The listing builds one solid part. Answer for the finished solid, in the listing's coordinates (mm). A direction names the side the tool comes from. Round coordinates to 2 decimals unless told otherwise and drop trailing zeros. Write each loop counter-clockwise with the first axis right and the second up, starting at its lowest first coordinate (ties: lowest second). Pieces come first, ordered by that corner, then holes. Notation, with made-up numbers: M 24,-21.5 L 70,-21.5 A10 ccw 70,-17.5 Z; hole C -33,4.25 d9. An arc over 180 degrees is marked long. One line per item, written item: value. Start each with the question number.
(1) Consider probe 1 along Y at (x, z) = (0, 4.75); probe 2 along Z at (x, y) = (3, -9.25); probe 3 along X at (y, z) = (0.25, 4). Determine where each line is inside the solid, lowest interval first.
(2) Given P1, Ø1.8, axis at x = 0, y = -0.5, coming from the +Z side; P2, Ø6, axis at y = 2, z = 5.5, coming from the -X side; P3, Ø5, axis at x = -7.5, z = 4, coming from the -Y side, each flat-ended and moving along its own axis, determine where each tip first touches the part or whether it passes through.
(3) Section B-B (z = 8.75) is taken. Determine the outline of the cut face in (x, y).
(4) For faces 1 (the flat face through (-2, -3, 10.5)), 2 (the flat face through (5, 0, 2)), determine the directions among +Z, -Z, +X, -X, +Y, -Y from which every point of the face is accessible in a straight line to the end or side of a thin tool.
(5) Section A-A (y = 0) is taken. Determine the outline of the cut face in (x, z).
(6) For a pull along Y with two mould halves and no side action, classify faces 3 (the cylindrical face through (-0.867, -3.905, 6.092)), 4 (the cylindrical face through (-3, 0, 6)), 5 (the flat face through (0, 0, 0)) as released by +Y, released by -Y, zero draft, split by the parting line, or undercut.
```python
from build123d import *

# Parameters (mm, degrees)
F0_R     = 11
F1_DEPTH = 2
F2_R     = 4
F2_R_2   = 3
F3_DEPTH = 8.5
F4_R     = 0.2
F5_SIZE  = 0.2


with BuildPart() as f1:
    # F0 (on Top) → F1 (new body)
    with BuildSketch(Plane.XY):
        Circle(F0_R)
    extrude(amount=F1_DEPTH)

    # F2 (on face) → F3 (join)
    with BuildSketch(Plane.XY.offset(2)):
        Circle(F2_R)
        Circle(F2_R_2, mode=Mode.SUBTRACT)
    extrude(amount=F3_DEPTH)

    # F4
    f4_edges = [f1.edges().sort_by_distance(p)[0] for p in [
        (-4, 0, 10.5),
        (-11, 0, 2),
        (-11, 0, 0),
    ]]
    fillet(f4_edges, radius=F4_R)

    # F5
    f5_edges = [f1.edges().sort_by_distance(p)[0] for p in [
        (-3, 0, 10.5),
    ]]
    chamfer(f5_edges, length=F5_SIZE)


solid = f1.part
```
Recorded:
1. probe 1: y = -4 to -3, 3 to 4
1. probe 2: z = 0 to 2
1. probe 3: x = -3.99 to -2.99, 2.99 to 3.99
2. P1: stops at z = 2
2. P2: stops at x = -4
2. P3: stops at y = -9.1
3. outline: C 0,0 d8; hole C 0,0 d6
4. face 1: +Z, +X, -X, +Y, -Y
4. face 2: +Z
5. outline: M -11,0.2 A0.2 ccw -10.8,0 L 10.8,0 A0.2 ccw 11,0.2 L 11,1.8 A0.2 ccw 10.8,2 L 4,2 L 4,10.3 A0.2 ccw 3.8,10.5 L 3.2,10.5 L 3,10.3 L 3,2 L -3,2 L -3,10.3 L -3.2,10.5 L -3.8,10.5 A0.2 ccw -4,10.3 L -4,2 L -10.8,2 A0.2 ccw -11,1.8 Z
6. face 3: split by the parting line
6. face 4: undercut
6. face 5: zero draft
